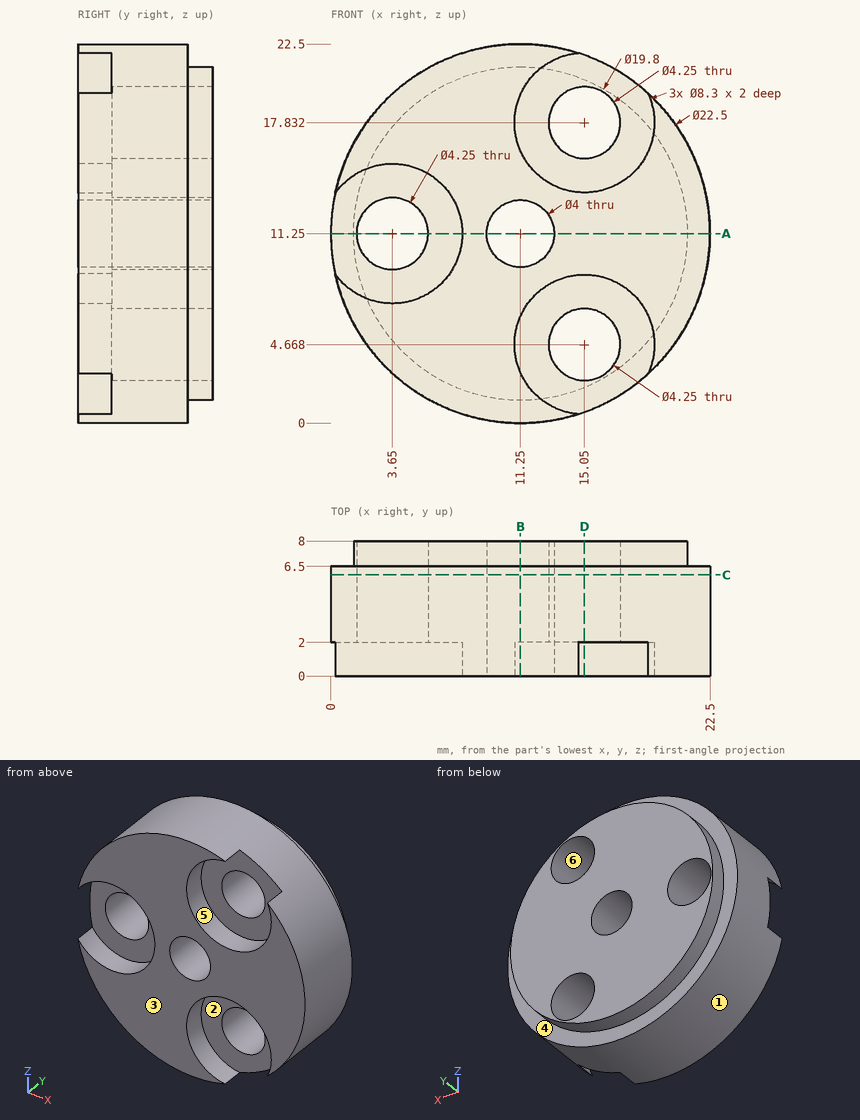
Could you check a few things on this drawing? It's one solid part, dimensions in mm from its lowest x, y, z. A direction names the side the tool comes from. Give positions to 0.01 mm unless a question says otherwise; leave off trailing zeros. Order: outer loops, then holes, each group sorted by start corner. A loop starts at its lowest first (then second) coordinate and runs counter-clockwise, first axis right, second up. Notation, with made-up numbers: (35.5, 82.25) -> (68.5, 82.25) arc R10 ccw to (68.5, 96.25) -> close; hole circle Ø7 at (-11, 89.5). An arc over 180 degrees is marked (long way). Answer in a Markdown table with one row per item. Add a question column.
Item 1: Please list where these lines run through material, in increasing order: probe 1 along X at (y, z) = (5, 11.25) (3 decimals); probe 2 along Z at (x, y) = (17, 7.5) (1 decimal); probe 3 along Z at (x, y) = (14.5, 5.25) (1 decimal).
Item 2: Imagine slicing it at B-B (x = 11.25). List the corners of the cut face in (y, z) for me.
Item 3: I'm going to push flat-ended pins straight in: P1, Ø5, axis at x = 15.05, z = 4.67, coming from the -Y side; P2, Ø3.5, axis at x = 3.65, z = 11.25, coming from the -Y side; P3, Ø3, axis at y = 7, z = 18, coming from the -X side; P4, Ø13.5, axis at x = 15.05, z = 4.67, coming from the +Y side. Where does each tip first touch, or does it pass through?
Item 4: Imagine slicing it at C-C (y = 6). Count the separate pieces of the cut face and the enclosed holes in it.
Item 5: We'd pull the mould along Z, two halves only. Please class the marked faces 1, 2 and 3: pulls with the +Z half, pulls with the -Z half, needs draft (parallel to the pull), parting line crosses it, or undercut.
Item 6: Imagine slicing it at A-A (z = 11.25). List the corners of the cut face in (x, y) for me (3 decimals), and give its area (3 significant figures).
Item 7: For the marked faces 4, 5 and 6, which set-ups out of +Z, -Z, +X, -X, +Y, -Y let a thin tool reach every point of the face, with its end or its side?
Item 8: Imagine slicing it at D-D (x = 15.05). List the corners of the cut face in (y, z) for me.
Result:
| question | item | result |
|---|---|---|
| 1 | probe 1 | 0 to 1.525, 5.775 to 9.25, 13.25 to 22.5 |
| 1 | probe 2 | 3.2 to 3.8, 5.5 to 17, 18.7 to 19.3 |
| 1 | probe 3 | 0.5 to 2.6, 6.7 to 15.8, 19.9 to 22 |
| 2 | outline | (0, 0) -> (6.5, 0) -> (6.5, 1.35) -> (8, 1.35) -> (8, 9.25) -> (0, 9.25) -> (0, 6.34) -> (2, 6.34) -> (2, 3) -> (0, 3) -> close; (0, 13.25) -> (8, 13.25) -> (8, 21.15) -> (6.5, 21.15) -> (6.5, 22.5) -> (0, 22.5) -> (0, 19.5) -> (2, 19.5) -> (2, 16.16) -> (0, 16.16) -> close |
| 3 | P1 | y = 2 |
| 3 | P2 | through |
| 3 | P3 | x = 1.35 |
| 3 | P4 | y = 8 |
| 4 | separate pieces | 1 |
| 4 | enclosed holes | 4 |
| 5 | face 1 | parting line crosses it |
| 5 | face 2 | undercut |
| 5 | face 3 | needs draft |
| 6 | outline | (0, 2) -> (1.525, 2) -> (1.525, 8) -> (1.35, 8) -> (1.35, 6.5) -> (0, 6.5) -> close; (5.775, 2) -> (7.8, 2) -> (7.8, 0) -> (9.25, 0) -> (9.25, 8) -> (5.775, 8) -> close; (13.25, 0) -> (22.5, 0) -> (22.5, 6.5) -> (21.15, 6.5) -> (21.15, 8) -> (13.25, 8) -> close |
| 6 | area | 103 mm2 |
| 7 | face 4 | +Y |
| 7 | face 5 | -Y |
| 7 | face 6 | +Y, -Y |
| 8 | outline | (0, 8.82) -> (2, 8.82) -> (2, 6.79) -> (8, 6.79) -> (8, 15.71) -> (2, 15.71) -> (2, 13.68) -> (0, 13.68) -> close; (2, 0.66) -> (6.5, 0.66) -> (6.5, 2.11) -> (8, 2.11) -> (8, 2.54) -> (2, 2.54) -> close; (2, 19.96) -> (8, 19.96) -> (8, 20.39) -> (6.5, 20.39) -> (6.5, 21.84) -> (2, 21.84) -> close |
